Read the model definition and answer for the solid it produces. Units are mm, in the model's axes. A direction names the side the tool comes from. Round coordinates to 2 decimals unless told otherwise and drop trailing zeros. Write each loop counter-clockwise with the first axis right and the second up, starting at its lowest first coordinate (ties: lowest second). Pieces come first, ordered by that corner, then holes. Notation, with made-up numbers: (43.5, -23) - (91.5, -23) arc R36 cw to (91.5, 16) - close; hole circle Ø4 at (79.25, 29). An arc over 180 degrees is marked (long way). Use one line per item in the form item = value. Start each with the question number.
1) The part is cut by section C-C, the plane z = 9.5. Give the vertices of the cut face in (x, y) (3 decimals).
2) Each of these flat-tipped pins is pushed along its axis until it touches: pin 1 (13 mm diameter, centred on x = 5, z = 13.5, fed in from -Y); pin 2 (2 mm diameter, centred on y = -27, z = 8, fed in from -X); pin 3 (5 mm diameter, centred on x = 5, z = 3.5, fed in from +Y); pin 4 (12 mm diameter, centred on x = 7, y = -32.5, fed in from +Z). Where does it stop, or does it pass through?
3) The part is cut by section A-A, the plane y = -18.5. Give the vertices of the cut face in (x, z) (3 decimals), plus the area to 3 significant figures.
4) The part is cut by section D-D, the plane x = 11.75. Give the vertices of the cut face in (y, z), plus the area to 3 significant figures.
5) The part is cut by section B-B, the plane x = 7. Give the vertices of the cut face in (y, z).
6) For faces 1 (the face through (4, -19, 18.298)), 2 (the face through (10, 0, 10)), 3 (the face through (18, -12.7, 8)), determine the directions among +Z, -Z, +X, -X, +Y, -Y from which every point of the face is accessible in a straight line to the end or side of a thin tool.
7) Consider line 1 along X through (y, z) = (-23.5, 13) (3 decimals); line 2 along Y through (x, z) = (9.75, 7); line 3 along Z through (x, y) = (10.75, -31.5). Determine where each line is inside the solid, lowest interval first. Write a range as from..to.
from build123d import *

# Parameters (mm, degrees)
F0_W     = 25.4
F0_H     = 6.35
F1_DEPTH = 38.1
F3_DEPTH = 12.7
F5_DEPTH = 12.7
F7_DEPTH = 12.7


with BuildPart() as f1:
    # F0 (on Front) → F1 (new body)
    with BuildSketch(Plane.XZ):
        with Locations((12.7, 3.175)):
            Rectangle(F0_W, F0_H)
        Polygon((0, 24.647629), (0, 6.35), (25.4, 6.35), align=None)
    extrude(amount=F1_DEPTH)

    # F2 (on face) → F3 (cut)
    with BuildSketch(Plane.XZ.offset(38.1)):
        Polygon((0, 6.35), (25.4, 6.35), (0, 24.647629), align=None)
    extrude(amount=-F3_DEPTH, mode=Mode.SUBTRACT)

    # F4 (on face) → F5 (cut)
    with BuildSketch(Plane.XZ.offset(25.4)):
        Polygon((8.814803, 18.297629), (0, 24.647629), (0, 18.297629), align=None)
    extrude(amount=-F5_DEPTH, mode=Mode.SUBTRACT)

    # F6 (on face) → F7 (cut)
    with BuildSketch(Plane.XZ.offset(25.4)):
        Polygon((15.875, 6.35), (25.4, 6.35), (15.875, 13.211611), align=None)
    extrude(amount=-F7_DEPTH, mode=Mode.SUBTRACT)


solid = f1.part
Geometry results:
q1.outline = (0, -25.4) - (15.875, -25.4) - (15.875, -12.7) - (21.027, -12.7) - (21.027, 0) - (0, 0) - close
q2.pin_1 = -25.4
q2.pin_2 = through
q2.pin_3 = 0
q2.pin_4 = 6.35
q3.outline = (0, 0) - (25.4, 0) - (25.4, 6.35) - (15.875, 6.35) - (15.875, 13.212) - (8.815, 18.298) - (0, 18.298) - close
q3.area = 333 mm2
q4.outline = (-38.1, 0) - (0, 0) - (0, 16.18) - (-25.4, 16.18) - (-25.4, 6.35) - (-38.1, 6.35) - close
q4.area = 492 mm2
q5.outline = (-38.1, 0) - (0, 0) - (0, 19.6) - (-12.7, 19.6) - (-12.7, 18.3) - (-25.4, 18.3) - (-25.4, 6.35) - (-38.1, 6.35) - close
q6.face_1 = +Z, +X, -X, -Y
q6.face_2 = +Z, -Z, +X, -X, +Y
q6.face_3 = +Z, +X, -Y
q7.line_1 = 0..15.875
q7.line_2 = -25.4..0
q7.line_3 = 0..6.35
